Read the model definition and answer for the solid it produces. Units are mm, in the model's axes. A direction names the side the tool comes from. Give positions to 0.01 mm unless a question says otherwise; leave off trailing zeros. Write each loop counter-clockwise with the first axis right and the second up, starting at its lowest first coordinate (ties: lowest second). Pieces come first, ordered by that corner, then holes.
```python
from build123d import *

# Parameters (mm, degrees)
F1_DEPTH = 30
F3_DEPTH = 40
F5_DEPTH = 50.6
F7_DEPTH = 72.9


with BuildPart() as f1:
    # F0 (on Front) → F1 (new body)
    with BuildSketch(Plane.XZ):
        Polygon((-55.277854, 10), (-65.277854, 0), (14.722146, 0), (4.722146, 10), (-5.277854, 10), (-5.277854, 40), (-45.277854, 40), (-45.277854, 10), align=None)
    extrude(amount=F1_DEPTH)

    # F2 (on Front) → F3 (join)
    with BuildSketch(Plane.XZ):
        with BuildLine():
            ThreePointArc((-45.065299, 40.219937), (-25.065299, 20.219937), (-5.065299, 40.219937))
            ThreePointArc((-5.065299, 40.219937), (-25.065299, 60.219937), (-45.065299, 40.219937))
        make_face()
    extrude(amount=F3_DEPTH)

    # F4 (on Front) → F5 (cut)
    with BuildSketch(Plane.XZ):
        with BuildLine():
            ThreePointArc((-35.12593, 40.110912), (-25.12593, 30.110912), (-15.12593, 40.110912))
            ThreePointArc((-15.12593, 40.110912), (-25.12593, 50.110912), (-35.12593, 40.110912))
        make_face()
    extrude(amount=F5_DEPTH, mode=Mode.SUBTRACT)

    # F6 (on Front) → F7 (cut)
    with BuildSketch(Plane.XZ):
        Polygon((-45.997363, 66.289328), (-45.592666, 40.134739), (-1.902011, 40.134739), (-3.919857, 66.289328), align=None)
    extrude(amount=F7_DEPTH, mode=Mode.SUBTRACT)


solid = f1.part
```
Item 1: Section D-D (z = 26) is taken. Write down the section's boundary in (x, y).
Result set:
outline: (-45.28, -30) - (-39.13, -30) - (-39.13, -40) - (-11, -40) - (-11, -30) - (-5.28, -30) - (-5.28, 0) - (-45.28, 0) - close
Item 2: Section A-A (z = 33.5) is taken. Write down the section's boundary in (x, y).
Result set:
outline: (-45.28, -30) - (-43.9, -30) - (-43.9, -40) - (-32.63, -40) - (-32.63, 0) - (-45.28, 0) - close; (-17.62, -40) - (-6.23, -40) - (-6.23, -30) - (-5.28, -30) - (-5.28, 0) - (-17.62, 0) - close
Item 3: Find the intervals of material crossed by line 1 along Y through (x, z) = (-44.5, 3.5); line 2 along X through (y, z) = (-9.5, 20); line 3 along Z through (x, y) = (-52.5, -19), in increasing order.
Result set:
line 1: y = -30 to 0
line 2: x = -45.28 to -5.28
line 3: z = 0 to 10
Item 4: Which of the six approach directions +Z, -Z, +X, -X, +Y, -Y give full straight-line access (tool end or side, diameter ignored) to faces 5 (the flat face through (-45.278, -15, 25)), 6 (the flat face through (-10, -20, 40.135))?
Result set:
face 5: +Z, -X, +Y, -Y
face 6: +Z, +X, -X, +Y, -Y
Item 5: Section C-C (x = -2.5) is taken. Write down the section's boundary in (y, z), and give its area (3 significant figures).
Result set:
outline: (-30, 0) - (0, 0) - (0, 10) - (-30, 10) - close
area: 300 mm2
Item 6: Determine the mould class of faces 1 (the flat face through (-25, -40, 28)), 2 (the flat face through (-60.21, -14.79, 5.07)), 3 (the flat face through (-5.278, -15, 23)), 4 (the flat face through (-26, -15, 0)) for opening direction Z: pulls with the +Z half, pulls with the -Z half, needs draft (parallel to the pull), parting line crosses it, or undercut.
Result set:
face 1: needs draft
face 2: pulls with the +Z half
face 3: undercut
face 4: pulls with the -Z half
Item 7: Each of these flat-tipped pins is pushed along its axis until it touches: pin 1 Ø2 at (y, z) = (-30.5, 14.5) entering from +X; pin 2 Ø3 at (x, y) = (-2.5, -20) entering from +Z; pin 3 Ø3 at (x, y) = (-23.5, -11.5) entering from +Z. Where does it stop, or does it pass through?
Result set:
pin 1: stops at x = -5.28
pin 2: stops at z = 10
pin 3: stops at z = 30.61
Item 8: Section B-B (y = -14) is taken. Write down the section's boundary in (x, z), and give its area (3 significant figures).
Result set:
outline: (-65.28, 0) - (14.72, 0) - (4.72, 10) - (-5.28, 10) - (-5.28, 37.31) arc R20 ccw to (-5.07, 40.13) - (-15.13, 40.13) arc R10 cw to (-35.13, 40.13) - (-45.07, 40.13) arc R20 ccw to (-45.06, 40) - (-45.28, 40) - (-45.28, 10) - (-55.28, 10) - close
area: 1,750 mm2
